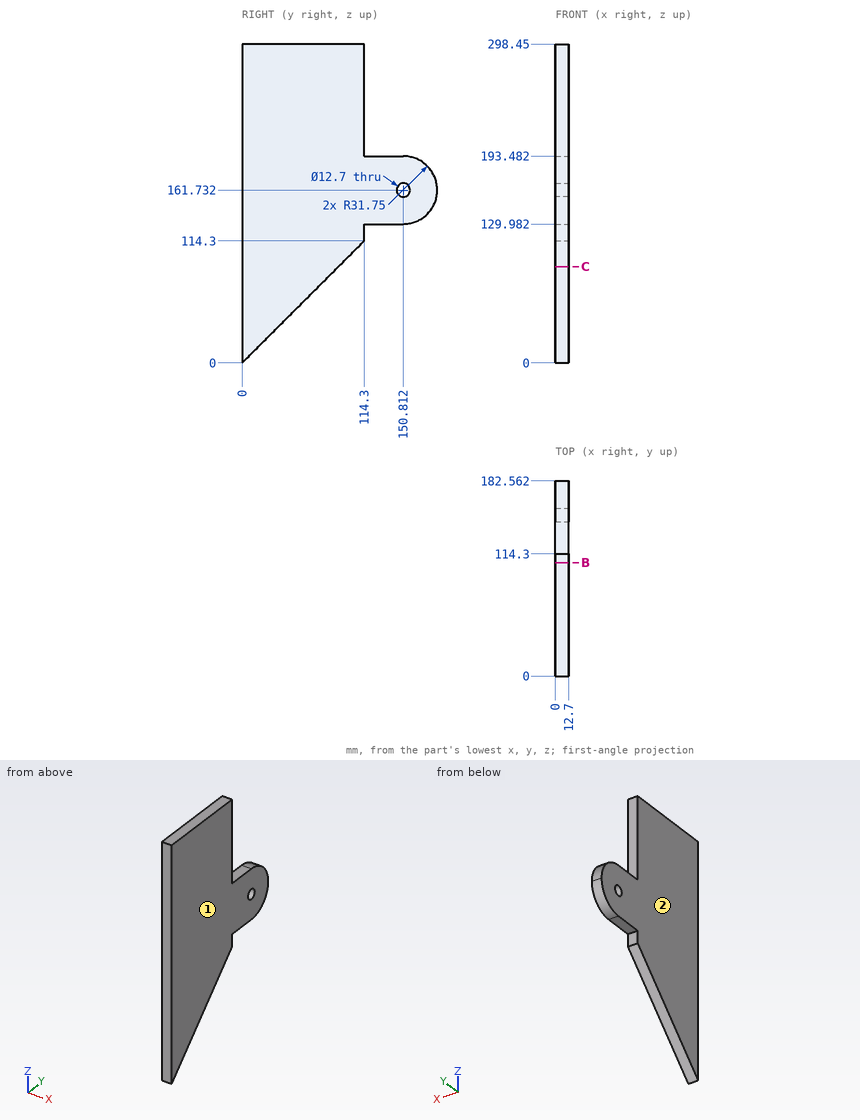
Design review of the part shown in the three views and the two pictorial views. Dimensions are in mm from the part's minimum x, y and z. Coordinates: 2 decimals unless noted, no trailing zeros. Loops run counter-clockwise (first coordinate to the right, second up) from the corner with the lowest first, then second, coordinate; pieces in that order, holes last.
(1) Consider section B-B, the plane y = 106. Give the boundary of the cut face in (x, z).
Determined:
outline: (0, 106) - (12.7, 106) - (12.7, 298.45) - (0, 298.45) - close
(2) Consider section C-C, the plane z = 90. Give the boundary of the cut face in (x, y).
Determined:
outline: (0, 0) - (12.7, 0) - (12.7, 90) - (0, 90) - close
(3) Draft analysis for pull direction X (two halves, no side actions). For the marked faces 1 and 2, state which applies: +X half, -X half, draft (parallel to the pull), parting line (faces both ways), or undercut.
Determined:
face 1: +X half
face 2: -X half
(4) Wall thickness on L1, parallel to Z at x = 8.5, y = 150.5 (1 decimal); L2, parallel to Y at x = 5.5, z = 123; L3, parallel to Z at x = 6, y = 118.5: over which ranges is each line inside the solid? List them lowest first.
Determined:
L1: z = 130 to 155.4, 168.1 to 193.5
L2: y = 0 to 114.3
L3: z = 129.98 to 193.48
(5) Insertion check: P1, Ø4, axis at x = 6, y = 90, coming from the -Z side; P2, Ø3, axis at x = 9.5, z = 242, coming from the +Y side; P3, Ø6.5, axis at x = 6, y = 130, coming from the +Z side. Each pin has a flat end and moves straight along its axis. Give the tip position at first contact, or say it passes through.
Determined:
P1: stops at z = 88
P2: stops at y = 114.3
P3: stops at z = 193.48
